Part print with two shaded views. Sizes in mm from the minimum x, y, z corner. A direction names the side the tool comes from. Give positions to 0.01 mm unless a question says otherwise; leave off trailing zeros. Write each loop counter-clockwise with the first axis right and the second up, starting at its lowest first coordinate (ties: lowest second). Pieces come first, ordered by that corner, then holes. Notation, with made-up numbers: (-32.75, 10) - (16.25, 10) arc R15 cw to (16.25, 36) - close; hole circle Ø5 at (81, -2.75). An arc over 180 degrees is marked (long way). Answer as a JSON object with one key per item and string values.
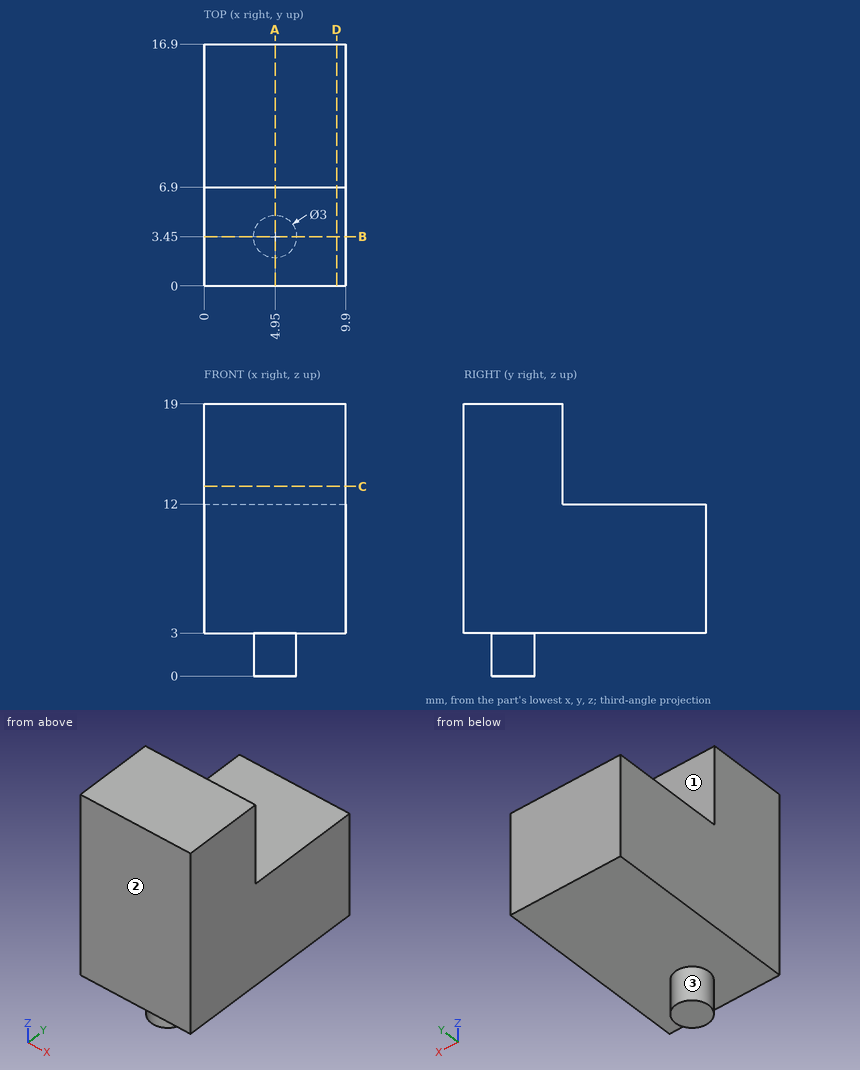
(1) Saw through at B-B, the plane y = 3.45. Give the cut face in (x, z), and give its area (3 significant figures).
Answer key:
{"outline": "(0, 3) - (3.45, 3) - (3.45, 0) - (6.45, 0) - (6.45, 3) - (9.9, 3) - (9.9, 19) - (0, 19) - close", "area": "167 mm²"}
(2) Flat gauge pins, fed straight in: P1, Ø1, axis at x = 4.5, z = 16, coming from the +Y side; P2, Ø3, axis at x = 6, y = 13.5, coming from the +Z side; P3, Ø3, axis at x = 4.5, y = 6.5, coming from the -Z side. Where does each tip first touch, or does it go through?
Answer key:
{"P1": "stops at y = 6.9", "P2": "stops at z = 12", "P3": "stops at z = 3"}
(3) Saw through at A-A, the plane x = 4.95. Give the cut face in (y, z), and give its area (3 significant figures).
Answer key:
{"outline": "(0, 3) - (1.95, 3) - (1.95, 0) - (4.95, 0) - (4.95, 3) - (16.9, 3) - (16.9, 12) - (6.9, 12) - (6.9, 19) - (0, 19) - close", "area": "209 mm²"}
(4) 3-axis set-ups, long thin cutter, end or side, ignore diameter. For the marked faces 1, 2 and 3: which of +Z, -Z, +X, -X, +Y, -Y reach the whole face in a straight line?
Answer key:
{"face 1": "+Z, +X, -X, +Y", "face 2": "+Z, -Z, +X, -X, -Y", "face 3": "-Z"}
(5) Saw through at C-C, the plane z = 13.25. Give the cut face in (x, y), and give its area (3 significant figures).
Answer key:
{"outline": "(0, 0) - (9.9, 0) - (9.9, 6.9) - (0, 6.9) - close", "area": "68.3 mm²"}
(6) Saw through at D-D, the plane x = 9.25. Give the cut face in (y, z).
Answer key:
{"outline": "(0, 3) - (16.9, 3) - (16.9, 12) - (6.9, 12) - (6.9, 19) - (0, 19) - close"}
(7) Probe L1, parallel to Z at x = 4.5, y = 9.5; L2, parallel to Z at x = 2, y = 1; L3, parallel to Y at x = 1.25, z = 16.5. List the from-to ranges inside material, lowest first. Write a range as [from, to].
Answer key:
{"L1": "z = [3, 12]", "L2": "z = [3, 19]", "L3": "y = [0, 6.9]"}
